Model file for the job. Use its own axes, mm. A direction names the side the tool comes from. Coordinates: 2 decimals unless noted, no trailing zeros. Loops run counter-clockwise (first coordinate to the right, second up) from the corner with the lowest first, then second, coordinate; pieces in that order, holes last.
from build123d import *

# Parameters (mm, degrees)
BOSS_EXTRUDE1_DEPTH = 2


with BuildPart() as part:
    # Sketch1 → Revolve1 (revolve)
    with BuildSketch(Plane.XY, mode=Mode.PRIVATE) as revolve1_sk:
        with BuildLine():
            Line((0, 11.475), (2.25, 11.475))
            ThreePointArc((2.25, 11.475), (2.603553391, 11.328553391), (2.75, 10.975))
            Line((2.75, 10.975), (2.75, 9.425))
            ThreePointArc((2.75, 9.425), (2.603553391, 9.071446609), (2.25, 8.925))
            Line((2.25, 8.925), (2.25, 8.525))
            Line((2.25, 8.525), (1.375, 8.525))
            Line((1.375, 8.525), (1.375, -11.475))
            Line((1.375, -11.475), (0, -11.475))
            Line((0, -11.475), (0, 11.475))
        make_face()
    revolve(revolve1_sk.sketch.rotate(Axis((0, 4.094224924, 0), (0, -1, 0)), 90), axis=Axis((0, 4.094224924, 0), (0, -1, 0)))


with BuildPart() as body_2:
    # Sketch2 → Boss-Extrude1 (new body)
    with BuildSketch(Plane(origin=(0, 11.475, 0), x_dir=(1, 0, 0), z_dir=(0, 1, 0))):
        Polygon((0, 1.443375673), (-1.25, 0.721687836), (-1.25, -0.721687836), (0, -1.443375673), (1.25, -0.721687836), (1.25, 0.721687836), align=None)
    extrude(amount=-BOSS_EXTRUDE1_DEPTH)

    # Sketch3 → Cut-Revolve1 (revolve, cut)
    with BuildSketch(Plane(origin=(0, 0, 0), x_dir=(0, 0, -1), z_dir=(1, 0, 0))):
        Polygon((0, 9.875), (0.4, 9.875), (1.443375673, 10.075), (1.443375673, 9.475), (0, 9.475), align=None)
    revolve(axis=Axis((0, 9.475, 0), (0, 1, 0)), mode=Mode.SUBTRACT)


with BuildPart() as part_1:
    add(part.part)

    # Combine1: cut body 2
    add(body_2.part, mode=Mode.SUBTRACT)


solid = part_1.part
Q1. Which spindle directions (+Z, -Z, +X, -X, +Y, -Y) get a long thin tool onto all of the face, cutting with end or side? Do faces 1 (the flat face through (0, -11.475, 0)), 2 (the cylindrical face through (-1.52, 8.72, -1.66)), 3 (the flat face through (-0.63, 10.77, 1.08)). Say none if no direction does.
Answers:
face 1: +Z, -Z, +X, -X, -Y
face 2: -Y
face 3: +Y
Q2. Flat gauge pins, fed straight in: P1, Ø1, axis at x = 0, y = -3.5, coming from the -Z side (3 decimals); P2, Ø1.5, axis at y = -2.5, z = -1, coming from the -X side; P3, Ø1, axis at x = 0, z = 0.5, coming from the +Y side. Where does each tip first touch, or does it go through?
Answers:
P1: stops at z = -1.375
P2: stops at x = -1.35
P3: stops at y = 9.99
Q3. Slice it at A-A (z = 0). List the corners of the cut face in (x, y) (3 decimals), and give its area (3 significant figures).
Answers:
outline: (-2.75, 9.425) arc R0.5 ccw to (-2.25, 8.925) - (-2.25, 8.525) - (-1.375, 8.525) - (-1.375, -11.475) - (1.375, -11.475) - (1.375, 8.525) - (2.25, 8.525) - (2.25, 8.925) arc R0.5 ccw to (2.75, 9.425) - (2.75, 10.975) arc R0.5 ccw to (2.25, 11.475) - (1.25, 11.475) - (1.25, 10.038) - (0.4, 9.875) - (-0.4, 9.875) - (-1.25, 10.038) - (-1.25, 11.475) - (-2.25, 11.475) arc R0.5 ccw to (-2.75, 10.975) - close
area: 66.7 mm2
Q4. Slice it at B-B (y = -7). List the corners of the cut face in (x, z) (3 decimals), and give its area (3 significant figures).
Answers:
outline: circle Ø2.75 at (0, 0)
area: 5.94 mm2
Q5. Drill centre lines: line 1 (Z direction, x = 0.5, y = 10.5); line 2 (Y direction, x = 1.85, z = 0.8) (3 decimals); line 3 (Z direction, x = -0.9, y = -9.25). Where is each one in solid material? Low to high.
Answers:
line 1: z = -2.7 to -1.15, 1.15 to 2.7
line 2: y = 8.525 to 11.475
line 3: z = -1.04 to 1.04
Q6. Mould opens along X. For faces 4 (the flat face through (1.5, 8.525, 0.5)), 5 (the cylindrical face through (1.34, -1.62, -0.3)), 6 (the flat face through (-0.616, 10.767, -1.088)) say: +X half, -X half, draft (parallel to the pull), parting line (faces both ways), or undercut.
Answers:
face 4: draft
face 5: parting line
face 6: undercut
